Read the model definition and answer for the solid it produces. Units are mm, in the model's axes. A direction names the side the tool comes from. Coordinates: 2 decimals unless noted, no trailing zeros. Loops run counter-clockwise (first coordinate to the right, second up) from the corner with the lowest first, then second, coordinate; pieces in that order, holes last. Notation, with made-up numbers: (-17.5, -25.75) -> (28.5, -25.75) arc R19 ccw to (28.5, -7.75) -> close; hole circle Ø8 at (-22, 43). An arc over 180 degrees is marked (long way). Answer in a Markdown table with one row per item.
```python
from build123d import *

# Parameters (mm, degrees)
MAINBASESKETCH_W          = 15.8
MAINBASESKETCH_H          = 3.2
MAINBASEEXTRUDE_DEPTH     = 7.9
STUDSSKETCH_R             = 2.4
STUDSEXTRUDE_DEPTH        = 1.6
STUDSPATTERN_COUNT        = 2
STUDSPATTERN_PITCH        = 8
STUDSPATTERN_COUNT_DIR2   = 2
STUDSPATTERN_PITCH_DIR2   = 8
MAINBASESHELL_T           = -1.2
UNDERSIDECIRCLEEXT_START  = -0.2
UNDERSIDECIRCLESKETCH_R   = 3.15
UNDERSIDECIRCLESKETCH_R_2 = 2.4
UNDERSIDECIRCLEEXT_DEPTH  = 1.6
SKETCH66_R                = 2.4
CUT_EXTRUDE19_DEPTH       = 24.398829954
CUT_EXTRUDE20_DEPTH       = 2.4
BOSS_EXTRUDE1_START       = -0.2
SKETCH66_6_R              = 3.25
SKETCH66_6_R_2            = 2.4
BOSS_EXTRUDE1_DEPTH       = 2.2


with BuildPart() as part:
    # MainBaseSketch → MainBaseExtrude (new, symmetric)
    with BuildSketch(Plane.XY):
        with Locations((8.581967213, 1.6)):
            Rectangle(MAINBASESKETCH_W, MAINBASESKETCH_H)
    extrude(amount=MAINBASEEXTRUDE_DEPTH, both=True)

    # StudsSketch → StudsExtrude (add)
    with BuildSketch(Plane(origin=(0, 3.2, 0), x_dir=(1, 0, 0), z_dir=(0, 1, 0))):
        with Locations((4.581967213, 4)):
            Circle(STUDSSKETCH_R)
    studsextrude = extrude(amount=STUDSEXTRUDE_DEPTH)

    # StudsPattern: StudsExtrude 2 × 2
    with Locations(*[(j * STUDSPATTERN_PITCH_DIR2, 0, i * STUDSPATTERN_PITCH) for i in range(STUDSPATTERN_COUNT) for j in range(STUDSPATTERN_COUNT_DIR2) if (i, j) != (0, 0)]):
        add(studsextrude)

    # MainBaseShell
    mainbaseshell_openings = [part.faces().sort_by_distance(p)[0] for p in [
        (8.581967213, 0, 0),
    ]]
    offset(amount=MAINBASESHELL_T, openings=mainbaseshell_openings, kind=Kind.INTERSECTION)

    # UnderSideCircleSketch → UnderSideCircleExt (add)
    with BuildSketch(Plane.XZ.offset(-2).offset(UNDERSIDECIRCLEEXT_START)):
        with Locations((8.581967213, 0)):
            Circle(UNDERSIDECIRCLESKETCH_R)
        with Locations((8.581967213, 0)):
            Circle(UNDERSIDECIRCLESKETCH_R_2, mode=Mode.SUBTRACT)
    extrude(amount=UNDERSIDECIRCLEEXT_DEPTH)

    # Sweep6: sweep along a curve in space
    with BuildLine() as sweep6_path:
        Line((16.481967213, 0, -7.9), (16.481967213, 3.2, -7.9))
    # Sketch64 → Sweep6 (sweep)
    with BuildSketch(Plane(origin=(0, 3.2, 0), x_dir=(1, 0, 0), z_dir=(0, 1, 0))):
        with BuildLine():
            Line((0.681967213, 7.9), (16.481967213, 7.9))
            ThreePointArc((16.481967213, 7.9), (14.174104013, 13.52161009), (8.581967213, 15.9))
            ThreePointArc((8.581967213, 15.9), (2.960357123, 13.550714964), (0.681967213, 7.9))
        make_face()
    sweep(path=sweep6_path.line)

    # Sketch66 → Cut-Extrude19 (cut, through all)
    with BuildSketch(Plane(origin=(0, 0, 0), x_dir=(-1, 0, 0), z_dir=(0, -1, 0))):
        with Locations(Location((-8.581967213, 12, 0), (0, 0, 90))):
            Circle(SKETCH66_R)
    extrude(amount=-CUT_EXTRUDE19_DEPTH, mode=Mode.SUBTRACT)

    # Sketch68 → Cut-Extrude20 (cut)
    with BuildSketch(Plane(origin=(0, 0, 0), x_dir=(-1, 0, 0), z_dir=(0, -1, 0))):
        with BuildLine():
            Line((-15.281967213, 7.9), (-1.881967213, 7.9))
            ThreePointArc((-1.881967213, 7.9), (-3.808255779, 12.873274015), (-8.581967213, 15.251450042))
            ThreePointArc((-8.581967213, 15.251450042), (-13.355678647, 12.873274015), (-15.281967213, 7.9))
        make_face()
    extrude(amount=-CUT_EXTRUDE20_DEPTH, mode=Mode.SUBTRACT)

    # Sketch66_6 → Boss-Extrude1 (add)
    with BuildSketch(Plane(origin=(0, 0, 0), x_dir=(-1, 0, 0), z_dir=(0, -1, 0)).offset(BOSS_EXTRUDE1_START)):
        with Locations((-8.581967213, 12)):
            Circle(SKETCH66_6_R)
        with Locations(Location((-8.581967213, 12, 0), (0, 0, 90))):
            Circle(SKETCH66_6_R_2, mode=Mode.SUBTRACT)
    extrude(amount=-BOSS_EXTRUDE1_DEPTH)


solid = part.part
```
1. A cutting plane is placed at C-C on z = 0. Give the vertices of the cut face in (x, y), and give its area (3 significant figures).
A:
| item | result |
|---|---|
| outline | (0.68, 0) -> (1.88, 0) -> (1.88, 2) -> (5.43, 2) -> (5.43, 0.6) -> (6.18, 0.6) -> (6.18, 2) -> (10.98, 2) -> (10.98, 0.6) -> (11.73, 0.6) -> (11.73, 2) -> (15.28, 2) -> (15.28, 0) -> (16.48, 0) -> (16.48, 3.2) -> (0.68, 3.2) -> close |
| area | 25.9 mm2 |
2. Given pin 1 Ø4.5 at (x, z) = (8.58, -12) entering from -Y; pin 2 Ø2 at (y, z) = (3.5, -6.5) entering from -X; pin 3 Ø4 at (x, z) = (4.58, -4) entering from -Y; pin 4 Ø0.6 at (x, y) = (11, 1) entering from -Z, each flat-ended and moving along its own axis, determine where each tip first touches the part or whether it passes through.
A:
| item | result |
|---|---|
| pin 1 | passes through |
| pin 2 | stops at x = 0.68 |
| pin 3 | stops at y = 2 |
| pin 4 | stops at z = -15.59 |
3. A cutting plane is placed at B-B on z = -10.25. Give the vertices of the cut face in (x, y).
A:
| item | result |
|---|---|
| outline | (1.01, 0) -> (2.27, 0) -> (2.27, 2.4) -> (5.84, 2.4) -> (5.84, 0.2) -> (6.94, 0.2) -> (6.94, 3.2) -> (1.01, 3.2) -> close; (10.22, 0.2) -> (11.32, 0.2) -> (11.32, 2.4) -> (14.9, 2.4) -> (14.9, 0) -> (16.13, 0) -> (16.13, 3.2) -> (10.22, 3.2) -> close |
4. Find the intervals of material crossed by probe 1 along X at (y, z) = (1.2, 0); probe 2 along X at (y, z) = (0.4, -14.5); probe 3 along Z at (x, y) = (14.25, 1.3), in increasing order.
A:
| item | result |
|---|---|
| probe 1 | x = 0.68 to 1.88, 5.43 to 6.18, 10.98 to 11.73, 15.28 to 16.48 |
| probe 2 | x = 4.09 to 5.96, 6.51 to 10.66, 11.21 to 13 |
| probe 3 | z = -13.44 to -11.66, -7.9 to -6.7, 6.7 to 7.9 |
5. A cutting plane is placed at A-A on y = 2.95. Give the vertices of the cut face in (x, z), and give its area (3 significant figures).
A:
| item | result |
|---|---|
| outline | (0.68, -7.9) arc R7.9 ccw to (8.58, -15.9) arc R8 ccw to (16.48, -7.9) -> (16.48, 7.9) -> (0.68, 7.9) -> close; hole circle Ø2.4 at (4.58, -4); hole circle Ø2.4 at (4.58, 4); hole circle Ø4.8 at (8.58, -12); hole circle Ø2.4 at (12.58, -4); hole circle Ø2.4 at (12.58, 4) |
| area | 313 mm2 |
6. A tool of negligible diameter and unlimited length cuts with its end or side. For faces 1 (the cylindrical face through (10.184, 3.989, 3.894)), 2 (the flat face through (5, 4.8, -4)), 3 (the cylindrical face through (13.69, 2.79, 4.46)), from which of +Z, -Z, +X, -X, +Y, -Y can it reach the whole face along a straight path? Write none if from no direction.
A:
| item | result |
|---|---|
| face 1 | +Y |
| face 2 | +Z, -Z, +X, -X, +Y |
| face 3 | -Y |
